Source: CAD feature listing. Evaluate the final solid. Frame: model axes, mm. Face numbers are marked on the shaded views. A direction names the side the tool comes from. Coordinates: 2 decimals unless noted, no trailing zeros. Write each loop counter-clockwise with the first axis right and the second up, starting at its lowest first coordinate (ties: lowest second). Pieces come first, ordered by that corner, then holes. Notation, with made-up numbers: (-16.5, -20) - (33.5, -20) arc R33 cw to (33.5, 18) - close; hole circle Ø9 at (-38, -39). An arc over 180 degrees is marked (long way). One line per item, written item: value.
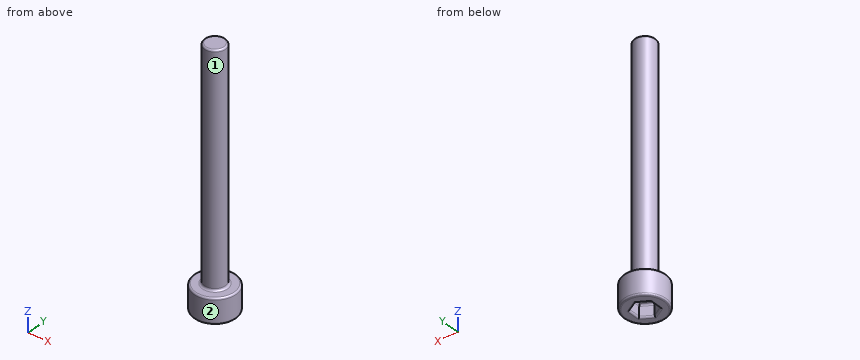
from build123d import *

# Parameters (mm, degrees)
SKETCH_1_R            = 5
EXTRUDE_490_DEPTH     = 6
SKETCH_2_R            = 2.5
EXTRUDE_581_DEPTH     = 54
CUT_EXTRUDE_774_DEPTH = 3
CHAMFER_830_SIZE2     = 0.4
CHAMFER_830_SIZE      = 0.230940108
FILLET_881_R          = 0.5
FILLET_2_R            = 0.4


with BuildPart() as part:
    # 草圖1 → Extrude 490 (new body)
    with BuildSketch(Plane.XY):
        Circle(SKETCH_1_R)
    extrude(amount=EXTRUDE_490_DEPTH)

    # 草圖2 → Extrude 581 (add)
    with BuildSketch(Plane.XY.offset(6)):
        Circle(SKETCH_2_R)
    extrude(amount=EXTRUDE_581_DEPTH)

    # 草圖3 → Cut-Extrude 774 (cut)
    with BuildSketch(Plane(origin=(0, 0, 0), x_dir=(-1, 0, 0), z_dir=(0, 0, -1))):
        Polygon((2.5, -1.443375673), (2.5, 1.443375673), (0, 2.886751346), (-2.5, 1.443375673), (-2.5, -1.443375673), (0, -2.886751346), align=None)
    extrude(amount=-CUT_EXTRUDE_774_DEPTH, mode=Mode.SUBTRACT)

    # Chamfer 830
    chamfer_830_edges = [part.edges().sort_by_distance(p)[0] for p in [
        (-5, 0, 0),
    ]]
    chamfer(chamfer_830_edges, length=CHAMFER_830_SIZE, length2=CHAMFER_830_SIZE2)

    # Fillet 881
    fillet_881_edges = [part.edges().sort_by_distance(p)[0] for p in [
        (-2.5, 0, 6),
    ]]
    fillet(fillet_881_edges, radius=FILLET_881_R)

    # 圓角2
    fillet_2_edges = [part.edges().sort_by_distance(p)[0] for p in [
        (-1.25, -2.165063509, 3),
        (1.25, -2.165063509, 3),
        (2.5, 0, 3),
        (1.25, 2.165063509, 3),
        (-1.25, 2.165063509, 3),
        (-2.5, 0, 3),
        (-1.25, -2.165063509, 0),
        (-2.5, 0, 0),
        (-1.25, 2.165063509, 0),
        (1.25, 2.165063509, 0),
        (2.5, 0, 0),
        (1.25, -2.165063509, 0),
        (-5, 0, 0.230940108),
        (-4.6, 0, 0),
        (-5, 0, 6),
        (-2.5, 0, 60),
    ]]
    fillet(fillet_2_edges, radius=FILLET_2_R)


solid = part.part
1) Contact query for flat-ended pins moving along their axis: P1, Ø1.5, axis at y = 1.5, z = 28, coming from the -X side; P2, Ø1, axis at x = -3, y = -3, coming from the +Z side; P3, Ø1, axis at x = 2, y = -1.5, coming from the -Z side. Output: stop coordinate, or through.
Values found:
P1: x = -2.38
P2: z = 6
P3: z = 0.01
2) Section query A-A on z = 7. Output: boundary loops of the cut face in (x, y).
Values found:
outline: circle Ø5 at (0, 0)
3) Material intervals for line 1 (Z direction, x = -3.75, y = 0.25); line 2 (Z direction, x = -0.75, y = -2); line 3 (Y direction, x = 1.5, z = 29), sorted ascending.
Values found:
line 1: 0 to 6
line 2: 3 to 60
line 3: -2 to 2
4) Reachability of the marked faces 1 and 2 from +Z, -Z, +X, -X, +Y, -Y: full face, straight path, thin tool, end or side. Return the list, or none.
Values found:
face 1: +Z
face 2: +Z, -Z
